from build123d import *

# Parameters (mm, degrees)
F0_W     = 482.6
F0_H     = 488.95
F0_W_2   = 266.7
F0_H_2   = 19.05
F1_DEPTH = 19.05
F2_DEPTH = 742.95
F3_DEPTH = 742.95
F4_R     = 10.16
F5_DEPTH = 127
F6_W     = 266.7
F6_H     = 193.675
F6_H_2   = 127
F6_H_3   = 76.2
F6_W_2   = 482.6
F7_DEPTH = 25.4
F8_W     = 25.4
F8_H     = 101.6
F9_DEPTH = 1104.901


with BuildPart() as f1:
    # F0 (on Top) → F1 (new body)
    with BuildSketch(Plane.XY):
        Polygon((265.602367, -235.660885), (265.602367, 253.289115), (246.552367, 253.289115), (246.552367, -235.660885), (246.552367, -254.710885), (265.602367, -254.710885), align=None)
        Polygon((551.352367, -254.710885), (551.352367, 253.289115), (532.302367, 253.289115), (532.302367, -235.660885), (532.302367, -254.710885), align=None)
        Polygon((-553.547633, 253.289115), (-553.547633, -267.410885), (564.052367, -267.410885), (564.052367, 253.289115), (551.352367, 253.289115), (551.352367, -254.710885), (532.302367, -254.710885), (265.602367, -254.710885), (246.552367, -254.710885), (-236.047633, -254.710885), (-255.097633, -254.710885), (-521.797633, -254.710885), (-540.847633, -254.710885), (-540.847633, 253.289115), align=None)
        with Locations((5.252367, 8.814115)):
            Rectangle(F0_W, F0_H)
        Polygon((-521.797633, 253.289115), (-540.847633, 253.289115), (-540.847633, -254.710885), (-521.797633, -254.710885), (-521.797633, -235.660885), align=None)
        with Locations((398.952367, 8.814115)):
            Rectangle(F0_W_2, F0_H)
        Polygon((-236.047633, 253.289115), (-255.097633, 253.289115), (-255.097633, -235.660885), (-255.097633, -254.710885), (-236.047633, -254.710885), (-236.047633, -235.660885), align=None)
        with Locations((-388.447633, 8.814115)):
            Rectangle(F0_W_2, F0_H)
        with Locations((-388.447633, -245.185885)):
            Rectangle(F0_W_2, F0_H_2)
        with Locations((5.252367, -245.185885)):
            Rectangle(F0_W, F0_H_2)
        with Locations((398.952367, -245.185885)):
            Rectangle(F0_W_2, F0_H_2)
    extrude(amount=F1_DEPTH)

    # F0 (on Top) → F2 (join)
    with BuildSketch(Plane.XY):
        Polygon((-521.797633, 253.289115), (-540.847633, 253.289115), (-540.847633, -254.710885), (-521.797633, -254.710885), (-521.797633, -235.660885), align=None)
        Polygon((-236.047633, 253.289115), (-255.097633, 253.289115), (-255.097633, -235.660885), (-255.097633, -254.710885), (-236.047633, -254.710885), (-236.047633, -235.660885), align=None)
        Polygon((265.602367, -235.660885), (265.602367, 253.289115), (246.552367, 253.289115), (246.552367, -235.660885), (246.552367, -254.710885), (265.602367, -254.710885), align=None)
        Polygon((551.352367, -254.710885), (551.352367, 253.289115), (532.302367, 253.289115), (532.302367, -235.660885), (532.302367, -254.710885), align=None)
    extrude(amount=-F2_DEPTH)

    # F0 (on Top) → F3 (join)
    with BuildSketch(Plane.XY):
        with Locations((-388.447633, -245.185885)):
            Rectangle(F0_W_2, F0_H_2)
        with Locations((398.952367, -245.185885)):
            Rectangle(F0_W_2, F0_H_2)
    extrude(amount=-F3_DEPTH)

    # F4
    f4_edges = [f1.edges().sort_by_distance(p)[0] for p in [
        (-553.547633, -7.060885, 19.05),
        (5.252367, -267.410885, 19.05),
        (564.052367, -7.060885, 19.05),
        (5.252367, 253.289115, 19.05),
    ]]
    fillet(f4_edges, radius=F4_R)

    # F0 (on Top) → F5 (join)
    with BuildSketch(Plane.XY):
        with Locations((5.252367, -245.185885)):
            Rectangle(F0_W, F0_H_2)
    extrude(amount=-F5_DEPTH)

    # F6 (on face) → F7 (cut)
    with BuildSketch(Plane.XZ.offset(254.710885)):
        with Locations((-388.447633, -595.3125)):
            Rectangle(F6_W, F6_H)
        with Locations((-388.447633, -376.2375)):
            Rectangle(F6_W, F6_H)
        with Locations((-388.447633, -190.5)):
            Rectangle(F6_W, F6_H_2)
        with Locations((-388.447633, -63.5)):
            Rectangle(F6_W, F6_H_3)
        with Locations((5.252367, -63.5)):
            Rectangle(F6_W_2, F6_H_3)
        with Locations((398.952367, -63.5)):
            Rectangle(F6_W, F6_H_3)
        with Locations((398.952367, -190.5)):
            Rectangle(F6_W, F6_H_2)
        with Locations((398.952367, -376.2375)):
            Rectangle(F6_W, F6_H)
        with Locations((398.952367, -595.3125)):
            Rectangle(F6_W, F6_H)
    extrude(amount=-F7_DEPTH, mode=Mode.SUBTRACT)

    # F8 (on face) → F9 (cut, through all)
    with BuildSketch(Plane.YZ.offset(551.352367)):
        with Locations((240.589115, -692.15)):
            Rectangle(F8_W, F8_H)
    extrude(amount=-F9_DEPTH, mode=Mode.SUBTRACT)


solid = f1.part
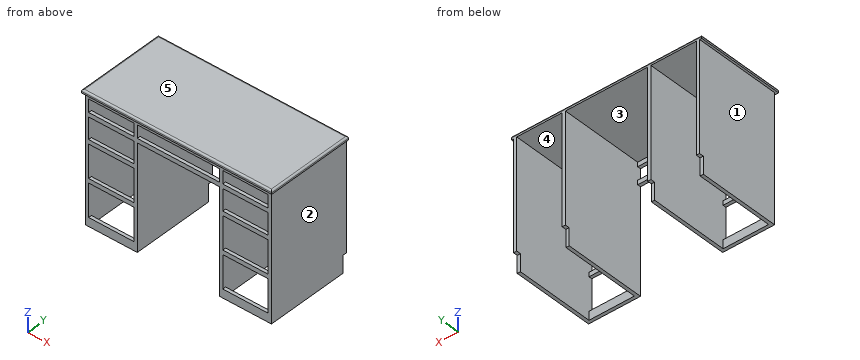
CAD build for the part. Positions are in the model's coordinates, mm. Face numbers are marked on the shaded views. A direction names the side the tool comes from. Coordinates: 2 decimals unless noted, no trailing zeros. Loops run counter-clockwise (first coordinate to the right, second up) from the corner with the lowest first, then second, coordinate; pieces in that order, holes last. Notation, with made-up numbers: (14, 62) - (61, 62) arc R10 ccw to (61, 80) - close; hole circle Ø7 at (-35, 15). An arc over 180 degrees is marked (long way). Write item = value, one per line. Start each with the question number.
Q1. Cut at D-D, the plane y = 23. List the corners of the cut face in (x, z), then the cut area to 3 significant figures.
Q2. Flat gauge pins, fed straight in: pin 1 Ø15 at (x, y) = (-249.5, 234.5) entering from -Z; pin 2 Ø1 at (y, z) = (-161.5, -157) entering from -X; pin 3 Ø1 at (y, z) = (-10.5, -105) entering from +X; pin 4 Ø4 at (x, z) = (-84.5, -126.5) entering from -Y. Where does each tip first touch, or does it go through?
Q3. Pull direction X, two halves, no side cores. Call the marked faces 1, 2 and 3: pulls with the +X half, pulls with the -X half, needs draft (parallel to the pull), parting line crosses it, or undercut.
Q4. Cut at C-C, the plane x = 414.5. List the corners of the cut face in (y, z) (3 decimals), then the cut area to 3 significant figures.
Q5. Drill centre lines: L1, parallel to X at y = 145, z = -33; L2, parallel to Z at x = 462.5, y = -244 (3 decimals); L3, parallel to Y at x = 371.5, z = -695.5. Where is each one in solid material? Low to high.
Q6. Cut at B-B, the plane z = -537. List the corners of the cut face in (x, y), then the cut area to 3 significant figures.
Q7. Which spindle directions (+Z, -Z, +X, -X, +Y, -Y) get a long thin tool onto all of the face, cutting with end or side? Do the marked faces 4 and 5. Say none if no direction does.
Q8. Cut at A-A, the plane x = 213.5. List the corners of the cut face in (y, z).
Computed:
q1.outline = (-553.55, 0) - (-540.85, 0) - (-540.85, -742.95) - (-521.8, -742.95) - (-521.8, 0) - (-255.1, 0) - (-255.1, -742.95) - (-236.05, -742.95) - (-236.05, 0) - (246.55, 0) - (246.55, -742.95) - (265.6, -742.95) - (265.6, 0) - (532.3, 0) - (532.3, -742.95) - (551.35, -742.95) - (551.35, 0) - (564.05, 0) - (564.05, 8.89) arc R10.16 ccw to (553.89, 19.05) - (-543.39, 19.05) arc R10.16 ccw to (-553.55, 8.89) - close
q1.area = 77,900 mm²
q2.pin_1 = -742.95
q2.pin_2 = -540.85
q2.pin_3 = 551.35
q2.pin_4 = -254.71
q3.face_1 = pulls with the -X half
q3.face_2 = pulls with the +X half
q3.face_3 = undercut
q4.outline = (-267.411, 0) - (-254.711, 0) - (-254.711, -25.4) - (-235.661, -25.4) - (-235.661, 0) - (253.289, 0) - (253.289, 8.89) arc R10.16 ccw to (243.129, 19.05) - (-257.251, 19.05) arc R10.16 ccw to (-267.411, 8.89) - close; (-254.711, -742.95) - (-235.661, -742.95) - (-235.661, -692.15) - (-254.711, -692.15) - close; (-254.711, -498.475) - (-235.661, -498.475) - (-235.661, -473.075) - (-254.711, -473.075) - close; (-254.711, -279.4) - (-235.661, -279.4) - (-235.661, -254) - (-254.711, -254) - close; (-254.711, -127) - (-235.661, -127) - (-235.661, -101.6) - (-254.711, -101.6) - close
q4.area = 12,800 mm²
q5.L1 = -540.85 to -521.8, -255.1 to -236.05, 246.55 to 265.6, 532.3 to 551.35
q5.L2 = -742.95 to -692.15, -498.475 to -473.075, -279.4 to -254, -127 to -101.6, -25.4 to 19.05
q5.L3 = -254.71 to -235.66
q6.outline = (-540.85, -254.71) - (-521.8, -254.71) - (-521.8, 253.29) - (-540.85, 253.29) - close; (-255.1, -254.71) - (-236.05, -254.71) - (-236.05, 253.29) - (-255.1, 253.29) - close; (246.55, -254.71) - (265.6, -254.71) - (265.6, 253.29) - (246.55, 253.29) - close; (532.3, -254.71) - (551.35, -254.71) - (551.35, 253.29) - (532.3, 253.29) - close
q6.area = 38,700 mm²
q7.face_4 = -Z, +Y
q7.face_5 = +Z, +X, -X, +Y, -Y
q8.outline = (-267.41, 0) - (-254.71, 0) - (-254.71, -25.4) - (-235.66, -25.4) - (-235.66, 0) - (253.29, 0) - (253.29, 8.89) arc R10.16 ccw to (243.13, 19.05) - (-257.25, 19.05) arc R10.16 ccw to (-267.41, 8.89) - close; (-254.71, -127) - (-235.66, -127) - (-235.66, -101.6) - (-254.71, -101.6) - close
